Read the model definition and answer for the solid it produces. Units are mm, in the model's axes. A direction names the side the tool comes from. Round coordinates to 2 decimals unless told otherwise and drop trailing zeros. Order: outer loops, then holes, each group sorted by start corner. A loop starts at its lowest first (then second) coordinate and runs counter-clockwise, first axis right, second up. Notation, with made-up numbers: (14, 12.5) -> (31, 12.5) arc R29 cw to (31, 44.5) -> close; hole circle Ø11 at (41, 29). An arc over 180 degrees is marked (long way). One line per item, written item: value. Start each with the question number.
1. Section A-A (x = -114.5) is taken. Give the vertices of the cut face in (y, z).
2. For faces 1 (the face through (145.49, 214.28, -4.93)), 2 (the face through (-88, 210, -5)), 3 (the face through (-292.482, 32.871, -4.93)), determine the directions among +Z, -Z, +X, -X, +Y, -Y from which every point of the face is accessible in a straight line to the end or side of a thin tool.
3. The mould has two halves that part along Y. Classify faces 4 (the face through (-115.49, 245.72, -4.93)), 5 (the face through (-28, 75, 0)), 6 (the face through (82.518, 47.129, -4.93)): released by +Y, released by -Y, zero draft, split by the parting line, or undercut.
4. Section C-C (y = 167) is taken. Give the vertices of the cut face in (x, z).
5. Flat-ended cylindrical pins translate along their axes: pin 1 Ø2 at (y, z) = (62, -6.5) entering from +X; pin 2 Ø1.5 at (y, z) = (74, -9) entering from -X; pin 3 Ø4 at (x, y) = (-62.5, 3.5) entering from +Z; pin 4 Ø5 at (y, z) = (112.5, -5) entering from +X. Find the tip coordinate at first contact, or state that the pin passes through.
6. Section B-B (z = -6.5) is taken. Give the vertices of the cut face in (x, y), then the cut area to 3 significant figures.
7. Section D-D (y = 205) is taken. Give the vertices of the cut face in (x, z).
8. Consider line 1 (Y direction, x = -97.5, z = -8.5); line 2 (X direction, y = 91.5, z = -5); line 3 (Y direction, x = -128.5, z = -5.25). Determine where each line is inside the solid, lowest interval first.
from build123d import *

# Parameters (mm, degrees)
F1_DEPTH = 10


with BuildPart() as f1:
    # F0 (on Top) → F1 (new body)
    with BuildSketch(Plane.XY):
        with BuildLine():
            Line((-70, 40), (-120, 40))
            Line((-120, 40), (-275, 40))
            ThreePointArc((-275, 40), (-292.67767, 32.67767), (-300, 15))
            Line((-300, 15), (-300, 0))
            Line((-300, 0), (-300, -15))
            ThreePointArc((-300, -15), (-292.67767, -32.67767), (-275, -40))
            Line((-275, -40), (125, -40))
            ThreePointArc((125, -40), (142.67767, -32.67767), (150, -15))
            Line((150, -15), (150, 15))
            ThreePointArc((150, 15), (142.67767, 32.67767), (125, 40))
            Line((125, 40), (100, 40))
            ThreePointArc((100, 40), (82.32233, 47.32233), (75, 65))
            Line((75, 65), (75, 185))
            ThreePointArc((75, 185), (82.32233, 202.67767), (100, 210))
            Line((100, 210), (135, 210))
            ThreePointArc((135, 210), (145.606602, 214.393398), (150, 225))
            Line((150, 225), (150, 235))
            ThreePointArc((150, 235), (145.606602, 245.606602), (135, 250))
            Line((135, 250), (-105, 250))
            ThreePointArc((-105, 250), (-115.606602, 245.606602), (-120, 235))
            Line((-120, 235), (-120, 225))
            ThreePointArc((-120, 225), (-115.606602, 214.393398), (-105, 210))
            Line((-105, 210), (-70, 210))
            ThreePointArc((-70, 210), (-52.32233, 202.67767), (-45, 185))
            Line((-45, 185), (-45, 65))
            ThreePointArc((-45, 65), (-52.32233, 47.32233), (-70, 40))
        make_face()
    extrude(amount=-F1_DEPTH)


solid = f1.part
Answer:
1. outline: (-40, -10) -> (40, -10) -> (40, 0) -> (-40, 0) -> close; (213.39, -10) -> (246.61, -10) -> (246.61, 0) -> (213.39, 0) -> close
2. face 1: +Z, -Z, +X
2. face 2: +Z, -Z, -X
2. face 3: +Z, -Z, -X, +Y
3. face 4: released by +Y
3. face 5: zero draft
3. face 6: undercut
4. outline: (-45, -10) -> (75, -10) -> (75, 0) -> (-45, 0) -> close
5. pin 1: x = 75.32
5. pin 2: x = -45
5. pin 3: z = 0
5. pin 4: x = 75
6. outline: (-300, -15) arc R25 ccw to (-275, -40) -> (125, -40) arc R25 ccw to (150, -15) -> (150, 15) arc R25 ccw to (125, 40) -> (100, 40) arc R25 cw to (75, 65) -> (75, 185) arc R25 cw to (100, 210) -> (135, 210) arc R15 ccw to (150, 225) -> (150, 235) arc R15 ccw to (135, 250) -> (-105, 250) arc R15 ccw to (-120, 235) -> (-120, 225) arc R15 ccw to (-105, 210) -> (-70, 210) arc R25 cw to (-45, 185) -> (-45, 65) arc R25 cw to (-70, 40) -> (-275, 40) arc R25 ccw to (-300, 15) -> close
6. area: 67,000 mm^2
7. outline: (-55, -10) -> (85, -10) -> (85, 0) -> (-55, 0) -> close
8. line 1: -40 to 40, 210 to 250
8. line 2: -45 to 75
8. line 3: -40 to 40
